Work out the finished part from the listing and answer in its coordinate system (mm). Coordinates: 2 decimals unless noted, no trailing zeros. Order: outer loops, then holes, each group sorted by start corner. A loop starts at its lowest first (then second) coordinate and runs counter-clockwise, first axis right, second up.
1. Determine the mould class of faces 1 (the flat face through (8, 2, 0)), 2 (the flat face through (0, 2, 5)), 3 (the cylindrical face through (-7.236, 2.465, 0.358)), 4 (the flat face through (0, 2, -5)) for opening direction Z: +Z half, -Z half, draft (parallel to the pull), parting line (faces both ways), or undercut.
2. The part is cut by section C-C, the plane y = 0.7. Give the vertices of the cut face in (x, z) (3 decimals), then the cut area to 3 significant figures.
3. The part is cut by section D-D, the plane x = 5. Give the vertices of the cut face in (y, z).
4. The part is cut by section B-B, the plane x = -6. Give the vertices of the cut face in (y, z), then the cut area to 3 significant figures.
5. The part is cut by section A-A, the plane z = 0. Give the vertices of the cut face in (x, y) (3 decimals).
6. Find the intervals of material crossed by probe 1 along X at (y, z) = (1.05, 0) (3 decimals); probe 2 along X at (y, z) = (4.45, 0.5); probe 3 along Z at (x, y) = (6.75, 1.4), in increasing order.
```python
from build123d import *

# Parameters (mm, degrees)
CROQUIS1_W              = 16
CROQUIS1_H              = 10
SALIENTE_EXTRUIR1_DEPTH = 5
CORTAR_EXTRUIR1_REACH   = 12.677
CROQUIS2_R              = 1.65


with BuildPart() as part:
    # Croquis1 → Saliente-Extruir1 (new body)
    with BuildSketch(Plane(origin=(0, 0, 0), x_dir=(1, 0, 0), z_dir=(0, 1, 0))):
        Rectangle(CROQUIS1_W, CROQUIS1_H)
    extrude(amount=SALIENTE_EXTRUIR1_DEPTH)

    # Croquis2 → Cortar-Extruir1 (cut, up to next)
    with BuildSketch(Plane.XZ, mode=Mode.PRIVATE) as cortar_extruir1_sk1:
        with Locations(Location((-5.625, 0, 0), (0, 0, 270))):
            Circle(CROQUIS2_R)
    cortar_extruir1_tool1 = extrude(cortar_extruir1_sk1.sketch, amount=-CORTAR_EXTRUIR1_REACH, mode=Mode.PRIVATE) & part.part
    # Croquis2 → Cortar-Extruir1 (cut, up to next)
    with BuildSketch(Plane.XZ, mode=Mode.PRIVATE) as cortar_extruir1_sk2:
        with Locations(Location((5.625, 0, 0), (0, 0, 270))):
            Circle(CROQUIS2_R)
    cortar_extruir1_tool2 = extrude(cortar_extruir1_sk2.sketch, amount=-CORTAR_EXTRUIR1_REACH, mode=Mode.PRIVATE) & part.part
    add(cortar_extruir1_tool1.solids().sort_by_distance((-5.625, 0, 0))[0], mode=Mode.SUBTRACT)
    add(cortar_extruir1_tool2.solids().sort_by_distance((5.625, 0, 0))[0], mode=Mode.SUBTRACT)


solid = part.part
```
Geometry says:
1. face 1: draft
1. face 2: +Z half
1. face 3: undercut
1. face 4: -Z half
2. outline: (-8, -5) - (8, -5) - (8, 5) - (-8, 5) - close; hole circle Ø3.3 at (-5.625, 0); hole circle Ø3.3 at (5.625, 0)
2. area: 143 mm2
3. outline: (0, -5) - (5, -5) - (5, -1.53) - (0, -1.53) - close; (0, 1.53) - (5, 1.53) - (5, 5) - (0, 5) - close
4. outline: (0, -5) - (5, -5) - (5, -1.61) - (0, -1.61) - close; (0, 1.61) - (5, 1.61) - (5, 5) - (0, 5) - close
4. area: 33.9 mm2
5. outline: (-8, 0) - (-7.275, 0) - (-7.275, 5) - (-8, 5) - close; (-3.975, 0) - (3.975, 0) - (3.975, 5) - (-3.975, 5) - close; (7.275, 0) - (8, 0) - (8, 5) - (7.275, 5) - close
6. probe 1: x = -8 to -7.275, -3.975 to 3.975, 7.275 to 8
6. probe 2: x = -8 to -7.2, -4.05 to 4.05, 7.2 to 8
6. probe 3: z = -5 to -1.21, 1.21 to 5
